Design review of the part built by this model. Coordinates are the model's own, in mm. A direction names the side the tool comes from. Coordinates: 2 decimals unless noted, no trailing zeros. Write each loop counter-clockwise with the first axis right and the second up, starting at its lowest first coordinate (ties: lowest second). Pieces come first, ordered by that corner, then holes.
Q1. Insertion check: pin 1 (2 mm diameter, centred on x = 397.5, y = -36.5, fed in from +Z); pin 2 (1 mm diameter, centred on x = -40.5, y = -20.5, fed in from -Z); pin 3 (3 mm diameter, centred on x = 145, z = 88.5, fed in from -Y); pin 4 (10 mm diameter, centred on x = -232, y = -2.5, fed in from -Z). Each pin has a flat end and moves straight along its axis. Give the tip position at first contact, or say it passes through.
Q2. For probe 1 along Y at (x, z) = (-60, -25.5); probe 2 along Y at (x, z) = (142, -8); probe 3 along Y at (x, z) = (131.5, 272.5), list the stretches that pass through material, from the lowest coordinate up.
Q3. Machinability: for faces 4 (the flat face through (-477.5, -44.3, 0.7)), 5 (the flat face through (-151.6, -3, 233.3)), 6 (the flat face through (72.11, -16.8, -1.42)), 7 (the flat face through (0, -44, -277)), which of the approach directions +Z, -Z, +X, -X, +Y, -Y give a long, thin tool a straight path to every point of the face, cutting with its end or side? Answer none if there is none.
Q4. Take a section at D-D (x = -9.5). Give the boundary of the cut face in (y, z).
Q5. Take a section at A-A (z = 402.5). Give the boundary of the cut face in (x, y).
Q6. Take a section at B-B (x = -134). Give the boundary of the cut face in (y, z).
Q7. Mouldability with a two-part tool opening along Z and no side actions: class faces 1 (the flat face through (-74.89, -18.66, -1.35)), 2 (the flat face through (-151.6, -3, -231.3)), 3 (the flat face through (-254.814, -25.308, -63.777)) as pulls with the +Z half, pulls with the -Z half, needs draft (parallel to the pull), parting line crosses it, or undercut.
```python
from build123d import *

# Parameters (mm, degrees)
SKETCH_1_W           = 1005
SKETCH_1_H           = 1080
EXTRUDE_1_DEPTH      = 3
EXTRUDE_2_DEPTH      = 515
EXTRUDE_2_DEPTH_BACK = 515
EXTRUDE_3_DEPTH      = 477.5
EXTRUDE_3_DEPTH_BACK = 477.5
SKETCH_5_W           = 1005
SKETCH_5_H           = 1080
SKETCH_5_W_2         = 975
SKETCH_5_H_2         = 1050
EXTRUDE_5_DEPTH      = 2


with BuildPart() as part:
    # Эскиз1 → Бобышка-Вытянуть1 (new body)
    with BuildSketch(Plane(origin=(0, 0, 0), x_dir=(1, 0, 0), z_dir=(0, 1, 0))):
        Rectangle(SKETCH_1_W, SKETCH_1_H)
    extrude(amount=EXTRUDE_1_DEPTH)

    # Эскиз2 → Бобышка-Вытянуть2 (add, two sides: drawn at the far end of the back side and taken through both)
    with BuildSketch(Plane.XY.offset(-EXTRUDE_2_DEPTH_BACK)):
        Polygon((25, -44), (-25, -44), (-101.210235533, 0), (-152.01408311, 0), (-152.01408311, -3), (-102.01408311, -3), (-25.803847577, -47), (25.803847577, -47), (102.01408311, -3), (152.01408311, -3), (152.01408311, 0), (101.210235533, 0), align=None)
    extrude(amount=EXTRUDE_2_DEPTH + EXTRUDE_2_DEPTH_BACK)

    # Эскиз3 → Бобышка-Вытянуть3 (add, two sides: drawn at the far end of the back side and taken through both)
    with BuildSketch(Plane(origin=(0, 0, 0), x_dir=(0, 0, -1), z_dir=(1, 0, 0)).offset(-EXTRUDE_3_DEPTH_BACK)):
        Polygon((-26.205771366, -47), (26.205771366, -47), (102.416006899, -3), (152.416006899, -3), (152.416006899, 0), (101.612159322, 0), (25.401923789, -44), (-25.401923789, -44), (-101.612159322, 0), (-152.416006899, 0), (-152.416006899, -3), (-102.416006899, -3), align=None)
    extrude(amount=EXTRUDE_3_DEPTH + EXTRUDE_3_DEPTH_BACK)

    # Эскиз5 → Бобышка-Вытянуть5 (add)
    with BuildSketch(Plane.XZ):
        Rectangle(SKETCH_5_W, SKETCH_5_H)
        Rectangle(SKETCH_5_W_2, SKETCH_5_H_2, mode=Mode.SUBTRACT)
    extrude(amount=EXTRUDE_5_DEPTH)


solid = part.part
```
Response:
1. pin 1: stops at z = 46.12
1. pin 2: stops at z = -72.97
1. pin 3: stops at y = -11.9
1. pin 4: stops at z = -540
2. probe 1: y = -47 to -43.94, -27.26 to -23.79, 0 to 3
2. probe 2: y = -47 to -44, -3 to 3
2. probe 3: y = -3 to 3
3. face 4: -Y
3. face 5: +Z, -X, -Y
3. face 6: none
3. face 7: -Z
4. outline: (-47, -515) - (-44, -515) - (-44, -31.4) - (-3, -102.42) - (-3, -152.42) - (0, -152.42) - (0, -525) - (-2, -525) - (-2, -540) - (3, -540) - (3, 540) - (-2, 540) - (-2, 525) - (0, 525) - (0, 152.42) - (-3, 152.42) - (-3, 102.42) - (-44, 31.4) - (-44, 515) - (-47, 515) - close; hole (-44, -25.4) - (0, -101.61) - (0, 101.61) - (-44, 25.4) - close
5. outline: (-502.5, -2) - (-487.5, -2) - (-487.5, 0) - (-152.01, 0) - (-152.01, -3) - (-102.01, -3) - (-25.8, -47) - (25.8, -47) - (102.01, -3) - (152.01, -3) - (152.01, 0) - (487.5, 0) - (487.5, -2) - (502.5, -2) - (502.5, 3) - (-502.5, 3) - close; hole (-101.21, 0) - (-25, -44) - (25, -44) - (101.21, 0) - close
6. outline: (-47, -26.21) - (-3, -102.42) - (-3, -515) - (0, -515) - (0, -525) - (-2, -525) - (-2, -540) - (3, -540) - (3, 540) - (-2, 540) - (-2, 525) - (0, 525) - (0, 515) - (-3, 515) - (-3, 102.42) - (-47, 26.21) - close; hole (-44, -25.4) - (-3, -96.42) - (-3, 96.42) - (-44, 25.4) - close
7. face 1: undercut
7. face 2: needs draft
7. face 3: pulls with the -Z half
